Source: CAD feature listing. Evaluate the final solid. Frame: model axes, mm. A direction names the side the tool comes from. Coordinates: 2 decimals unless noted, no trailing zeros. Order: outer loops, then holes, each group sorted by start corner. A loop starts at its lowest first (then second) coordinate and runs counter-clockwise, first axis right, second up.
Autodesk Inventor part; units mm, degrees
ref_plane "YZ Plane" through (0, 0, 0) normal (1, 0, 0) x (0, 1, 0)
ref_plane "XZ Plane" through (0, 0, 0) normal (0, 1, 0) x (-1, 0, 0)
ref_plane "XY Plane" through (0, 0, 0) normal (0, 0, 1) x (1, 0, 0)
sketch "Sketch1" plane through (0, 0, 0) normal (0, 0, 1) x (1, 0, 0)
  line L0 (-20.9848, 52.6481) -> (-30.7638, 52.6481)
  line L1 (-30.7638, 20.8981) -> (-30.7638, 52.6481)
  line L2 (-20.9848, 20.8981) -> (-30.7638, 20.8981)
  line L3 (-20.9848, 52.6481) -> (-20.9848, 20.8981)
  line L4 (-22.6993, 26.2773) -> (-22.6993, 24.127)
  line L5 (-22.6993, 24.127) -> (-29.0493, 24.127)
  line L6 (-29.0493, 24.127) -> (-29.0493, 26.2773)
  line L7 (-29.0493, 26.2773) -> (-22.6993, 26.2773)
  line L8 (-22.6993, 32.7351) -> (-22.6993, 30.5848)
  line L9 (-22.6993, 30.5848) -> (-29.0493, 30.5848)
  line L10 (-29.0493, 30.5848) -> (-29.0493, 32.7351)
  line L11 (-29.0493, 32.7351) -> (-22.6993, 32.7351)
  line L12 (-22.6993, 39.1928) -> (-22.6993, 37.0425)
  line L13 (-22.6993, 37.0425) -> (-29.0493, 37.0425)
  line L14 (-29.0493, 37.0425) -> (-29.0493, 39.1928)
  line L15 (-29.0493, 39.1928) -> (-22.6993, 39.1928)
  line L16 (-22.6993, 45.6505) -> (-22.6993, 43.5002)
  line L17 (-22.6993, 43.5002) -> (-29.0493, 43.5002)
  line L18 (-29.0493, 43.5002) -> (-29.0493, 45.6505)
  line L19 (-29.0493, 45.6505) -> (-22.6993, 45.6505)
  line L20 (-22.6993, 52.1083) -> (-22.6993, 49.958)
  line L21 (-22.6993, 49.958) -> (-29.0493, 49.958)
  line L22 (-29.0493, 49.958) -> (-29.0493, 52.1083)
  line L23 (-29.0493, 52.1083) -> (-22.6993, 52.1083)
  line L24 (-22.6993, 48.8794) -> (-22.6993, 46.7291)
  line L25 (-22.6993, 46.7291) -> (-29.0493, 46.7291)
  line L26 (-29.0493, 46.7291) -> (-29.0493, 48.8794)
  line L27 (-29.0493, 48.8794) -> (-22.6993, 48.8794)
  line L28 (-22.6993, 42.4217) -> (-22.6993, 40.2714)
  line L29 (-22.6993, 40.2714) -> (-29.0493, 40.2714)
  line L30 (-29.0493, 40.2714) -> (-29.0493, 42.4217)
  line L31 (-29.0493, 42.4217) -> (-22.6993, 42.4217)
  line L32 (-22.6993, 35.9639) -> (-22.6993, 33.8136)
  line L33 (-22.6993, 33.8136) -> (-29.0493, 33.8136)
  line L34 (-29.0493, 33.8136) -> (-29.0493, 35.9639)
  line L35 (-29.0493, 35.9639) -> (-22.6993, 35.9639)
  line L36 (-22.6993, 29.5062) -> (-22.6993, 27.3559)
  line L37 (-22.6993, 27.3559) -> (-29.0493, 27.3559)
  line L38 (-29.0493, 27.3559) -> (-29.0493, 29.5062)
  line L39 (-29.0493, 29.5062) -> (-22.6993, 29.5062)
  line L40 (-22.6993, 23.0485) -> (-22.6993, 20.8982)
  line L41 (-22.6993, 20.8982) -> (-29.0493, 20.8982)
  line L42 (-29.0493, 20.8982) -> (-29.0493, 23.0485)
  line L43 (-29.0493, 23.0485) -> (-22.6993, 23.0485)
  line L44 (-20.9848, 20.8981) -> (-20.4848, 20.8981)
  line L45 (-20.4848, 20.8981) -> (-30.7638, 20.8981)
  line L46 (-30.7638, 20.8981) -> (-31.2638, 20.8981)
  line L47 (-30.7638, 20.8981) -> (-30.7638, 24.7081)
  line L48 (-30.8638, 52.6481) -> (-20.7348, 52.6481)
  line L49 (-20.7348, 52.6481) -> (-20.4848, 24.7081)
  line L50 (-20.4848, 24.7081) -> (-30.8638, 24.7081)
  line L51 (-30.8638, 24.7081) -> (-31.2638, 24.7081)
  line L52 (-31.2638, 24.7081) -> (-31.2638, 52.6481)
  line L53 (-31.2638, 52.6481) -> (-20.7348, 52.6481)
  point P0 (0, 0)
  dimension "d0" = 0.5
  dimension "d1" = 0.5
extrude "Extrusion1" add sketch "Sketch1" along normal blind 12.41 contours L3 L50 L4 L7 L6 L1 L0 | L48 L49 L50 L3 | L1 L50 L51 L52 L53 L48 | L50 L6 L7 L4 | L8 L9 L10 L11 | L12 L13 L14 L15 | L16 L17 L18 L19 | L20 L21 L22 L23 | L24 L25 L26 L27 | L28 L29 L30 L31 | L32 L33 L34 L35 | L36 L37 L38 L39
sketch "Sketch2" plane through (-31.2638, 24.7081, 0) normal (-1, 0, 0) x (0, 0, 1)
  line L0 (12.41, 1.27) -> (22.57, 1.27)
  line L1 (12.41, 1.27) -> (0, 1.27)
  line L2 (0, 1.27) -> (0, 4.27)
  line L3 (0, 4.27) -> (12.41, 4.27)
  line L4 (12.41, 4.27) -> (12.41, 1.27)
  line L5 (0, 0) -> (12.41, 0)
  line L6 (12.41, 0) -> (0, 0)
  line L7 (0, 0) -> (0, 1.27)
  line L8 (0, 1.27) -> (12.41, 1.27)
  line L9 (12.41, 1.27) -> (12.41, 0)
  point P0 (0, -24.7081)
  dimension "d4" = 3
extrude "Extrusion2" cut sketch "Sketch2" against normal blind 12.41
sketch "Sketch3" plane through (-31.2638, 52.6481, 0) normal (-1, 0, 0) x (0, 0, 1)
  line L0 (25.999, 0) -> (12.41, 0)
  line L1 (12.41, -26.67) -> (12.41, 0)
  line L2 (12.41, -26.67) -> (22.57, -26.67)
  line L3 (22.57, -26.67) -> (22.57, -27.94)
  line L4 (22.57, -27.94) -> (12.41, -27.94)
  line L5 (12.41, -31.75) -> (12.41, -27.94)
  line L6 (25.999, -31.75) -> (12.41, -31.75)
  line L7 (25.999, -31.75) -> (25.999, 0)
  line L8 (0, -23.67) -> (12.41, -23.67)
  line L9 (12.41, 0) -> (12.41, -23.67)
  line L10 (0, 0) -> (12.41, 0)
  line L11 (0, 0) -> (0, -23.67)
  line L12 (0, 0) -> (25.999, 0)
  line L13 (25.999, 0) -> (25.999, -23.67)
  line L14 (25.999, -23.67) -> (0, -23.67)
  line L15 (0, -23.67) -> (0, 0)
  point P0 (0, -52.6481)
extrude "Extrusion3" add sketch "Sketch3" along normal blind 3 contours L7 L14 L1 L0 | L1 L8 L11 L10
sketch "Sketch4" plane through (-20.7348, 52.6481, 12.41) normal (1, 0.0089, 0) x (0, 0, -1)
  line L0 (0, -23.6709) -> (12.41, -23.6709)
  line L1 (12.41, -23.6709) -> (12.41, 0)
  line L2 (12.41, 0) -> (0, 0)
  line L3 (0, -23.6709) -> (0, 0)
  line L4 (0, 0.0022) -> (-13.589, 0.0022)
  line L5 (-13.589, 0.0022) -> (-13.589, -31.7465)
  line L6 (-13.589, -31.7465) -> (0, -31.7465)
  line L7 (0, -27.9366) -> (0, -31.7465)
  line L8 (0, -27.9366) -> (-10.16, -27.9366)
  line L9 (-10.16, -27.9366) -> (-10.16, -26.6667)
  line L10 (-10.16, -26.6667) -> (0, -26.6667)
  line L11 (0, 0.0022) -> (0, -26.6667)
  line L12 (0, -23.6709) -> (12.41, -23.6709)
  line L13 (-13.589, 0.0022) -> (12.41, 0.0022)
  line L14 (12.41, 0.0022) -> (12.41, -23.6709)
  line L15 (12.41, -23.6709) -> (-13.589, -23.6709)
  line L16 (-13.589, -23.6709) -> (-13.589, 0.0022)
  point P0 (12.41, -52.8315)
extrude "Extrusion4" add sketch "Sketch4" along normal blind 3 contours L3 L2 L1 L0 | L15 L5 L4 L11 L3 | L11 L13 L14 L2
properties part number "Guide"
1. Section query A-A on z = 16.5. Return loops of the section in (x, y), plus the area to 3 significant figures.
Findings:
outline: (-34.26, 28.98) - (-31.26, 28.98) - (-31.26, 52.65) - (-34.26, 52.65) - close; (-20.73, 52.65) - (-20.52, 28.98) - (-17.52, 29) - (-17.73, 52.68) - close
area: 142 mm2
2. Pin query (flat end, axial travel): P1, Ø8, axis at x = -30.5, z = 9.5, coming from the +Y side; P2, Ø7, axis at y = 36, z = 18.5, coming from the +X side; P3, Ø6, axis at y = 34.5, z = 7.5, coming from the +X side. Return the tip coordinate at first contact, or that it passes through.
Findings:
P1: stops at y = 52.65
P2: stops at x = -17.56
P3: stops at x = -17.55
3. Section query D-D on y = 48.75. Return loops of the section in (x, z), plus the area to 3 significant figures.
Findings:
outline: (-34.26, 0) - (-17.7, 0) - (-17.7, 26) - (-20.7, 26) - (-20.7, 12.41) - (-31.26, 12.41) - (-31.26, 26) - (-34.26, 26) - close
area: 287 mm2
4. Draft query along X for faces 3 (the face through (-34.264, 41, 13)), 4 (the face through (-29, 28.978, 7)), 5 (the face through (-31.264, 41, 19)). Return one class per face: released by +X, released by -X, zero draft, split by the parting line, or undercut.
Findings:
face 3: released by -X
face 4: zero draft
face 5: undercut
5. Ray query, line 1 (Z direction, x = -29, y = 48.75); line 2 (Y direction, x = -29.5, z = 7); line 3 (X direction, y = 30.5, z = 17). Return the intervals inside material, ascending.
Findings:
line 1: z = 0 to 12.41
line 2: y = 28.98 to 52.65
line 3: x = -34.26 to -31.26, -20.54 to -17.54
6. Section query C-C on x = -27.75. Return loops of the section in (y, z), plus the area to 3 significant figures.
Findings:
outline: (28.98, 0) - (52.65, 0) - (52.65, 12.41) - (28.98, 12.41) - close
area: 294 mm2
7. Access query for faces 1 (the face through (-26, 41, 0)), 2 (the face through (-29, 52.648, 7)). Directions: +Z, -Z, +X, -X, +Y, -Y. A direction counts if a zero-diameter tool reaches every point of the face in a straight line with its end or side. Return the directions, or none.
Findings:
face 1: -Z, +X, -X, +Y, -Y
face 2: +Z, -Z, -X, +Y
8. Section query B-B on y = 31.25. Return loops of the section in (x, z), plus the area to 3 significant figures.
Findings:
outline: (-34.26, 0) - (-17.54, 0) - (-17.54, 26) - (-20.54, 26) - (-20.54, 12.41) - (-31.26, 12.41) - (-31.26, 26) - (-34.26, 26) - close
area: 289 mm2
